```python
from build123d import *

# Parameters (mm, degrees)
EXTRUDE_1_DEPTH          = 35
SKETCH_4_W               = 45
SKETCH_4_H               = 5
CUT_EXTRUDE_1_DEPTH      = 8
CUT_EXTRUDE_2_DEPTH      = 189.679622641
CUT_EXTRUDE_3_DEPTH      = 166.90660023
CUT_EXTRUDE_3_DEPTH_BACK = 166.90660023
SKETCH_6_R               = 11
CHAMFER_1_SIZE           = 2
CHAMFER_2_SIZE           = 3


with BuildPart() as part:
    # Эскиз1 → Повернуть1 (revolve)
    with BuildSketch(Plane.XY, mode=Mode.PRIVATE) as revolve_1_sk:
        Polygon((0, 0), (0, 27.5), (80, 27.5), (80, 40), (145, 40), (145, 0), align=None)
    revolve(revolve_1_sk.sketch.rotate(Axis((0, 0, 0), (-1, 0, 0)), 90), axis=Axis((0, 0, 0), (-1, 0, 0)))

    # Эскиз3 → Бобышка-Вытянуть1 (add)
    with BuildSketch(Plane.ZY):
        Polygon((0, -15.556349186), (-15.556349186, 0), (0, 15.556349186), (15.556349186, 0), align=None)
    extrude(amount=EXTRUDE_1_DEPTH)

    # Эскиз4 → Вырез-Вытянуть1 (cut, symmetric)
    with BuildSketch(Plane(origin=(0, 0, 0), x_dir=(1, 0, 0), z_dir=(0, 1, 0))):
        with Locations((37.5, 25)):
            Rectangle(SKETCH_4_W, SKETCH_4_H)
    extrude(amount=CUT_EXTRUDE_1_DEPTH, both=True, mode=Mode.SUBTRACT)

    # Эскиз5 → Вырез-Вытянуть2 (cut, symmetric)
    with BuildSketch(Plane(origin=(145, 0, 0), x_dir=(0, 0, -1), z_dir=(1, 0, 0))):
        Polygon((-220.667748268, 35), (-19.364916731, 35), (19.364916731, 35), (220.667748268, 35), (220.667748268, 437.605663073), (-220.667748268, 437.605663073), align=None)
    cut_extrude_2 = extrude(amount=CUT_EXTRUDE_2_DEPTH, both=True, mode=Mode.SUBTRACT)

    # Зеркальное отражение1: Вырез-Вытянуть2 across plane
    add(cut_extrude_2.mirror(Plane.ZX), mode=Mode.SUBTRACT)

    # Эскиз6 → Вырез-Вытянуть3 (cut, two sides: drawn at the far end of the back side and taken through both)
    with BuildSketch(Plane(origin=(0, 35, 0), x_dir=(1, 0, 0), z_dir=(0, 1, 0)).offset(-CUT_EXTRUDE_3_DEPTH_BACK)):
        with Locations(Location((112.5, 0, 0), (0, 0, 270))):
            Circle(SKETCH_6_R)
    extrude(amount=CUT_EXTRUDE_3_DEPTH + CUT_EXTRUDE_3_DEPTH_BACK, mode=Mode.SUBTRACT)

    # Фаска1
    chamfer_1_edges = [part.edges().sort_by_distance(p)[0] for p in [
        (145, 0, -40),
        (80, 0, -40),
    ]]
    chamfer(chamfer_1_edges, length=CHAMFER_1_SIZE)

    # Фаска2
    chamfer_2_edges = [part.edges().sort_by_distance(p)[0] for p in [
        (0, 0, 27.5),
    ]]
    chamfer(chamfer_2_edges, length=CHAMFER_2_SIZE)


solid = part.part
```
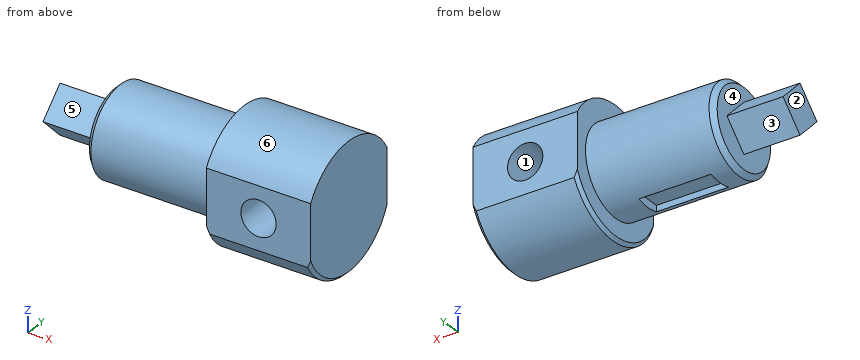
The model under review builds one solid part; all positions refer to its coordinate system, in mm. Face numbers are marked on the shaded views. A direction names the side the tool comes from. Coordinates: 2 decimals unless noted, no trailing zeros. Write each loop counter-clockwise with the first axis right and the second up, starting at its lowest first coordinate (ties: lowest second). Pieces come first, ordered by that corner, then holes. Notation, with made-up numbers: (32.5, -23) -> (61.5, -23) arc R10 cw to (61.5, -19) -> close; hole circle Ø6 at (29.5, 18). An arc over 180 degrees is marked (long way). One line per item, written item: value. Start each with the question number.
Q1. To check wall thickness, follow probe 1 along X at (y, z) = (2.5, 0); probe 2 along X at (y, z) = (-20, 0); probe 3 along Z at (x, y) = (112, -1). State the ranges of each line that lie inside material, in increasing order.
Q2. The part is to be moulded in two halves that separate along X. For the marked faces 1, 2 and 3, say which applies: +X half, -X half, draft (parallel to the pull), parting line (faces both ways), or undercut.
Q3. Add section B-B, the plane x = -9.5. Give the boundary of the cut face in (y, z).
Q4. For the marked faces 4, 5 and 6, list the 3-axis set-ups (+Z, -Z, +X, -X, +Y, -Y) from which the entire face can be reached by the end or side of a thin tool; tool diameter is ignored.
Q5. Clearance check with flat-ended pins moving along their axes: P1, Ø4, axis at x = 100.5, y = -20, coming from the -Z side; P2, Ø1, axis at x = 2.5, z = -13.5, coming from the -Y side; P3, Ø1.5, axis at x = 111.5, y = -6, coming from the -Z side. State where each tip first meets the part, or that it passes through.
Q6. Add section A-A, the plane x = 112.5. Give the boundary of the cut face in (y, z).
Response:
1. probe 1: -35 to 101.5, 123.5 to 145
1. probe 2: 0 to 101.5, 123.5 to 145
1. probe 3: -39.99 to -10.99, 10.99 to 39.99
2. face 1: undercut
2. face 2: -X half
2. face 3: draft
3. outline: (-15.56, 0) -> (0, -15.56) -> (15.56, 0) -> (0, 15.56) -> close
4. face 4: -X
4. face 5: +Z, -X, -Y
4. face 6: +Z, +X, -X
5. P1: z = -35.72
5. P2: y = -24.02
5. P3: z = -39.65
6. outline: (-35, -19.36) arc R40 ccw to (35, -19.36) -> (35, -11) -> (-35, -11) -> close; (-35, 11) -> (35, 11) -> (35, 19.36) arc R40 ccw to (-35, 19.36) -> close
